Can you work these out from the model? Positions are in its coordinate system, mm. A direction names the side the tool comes from. Coordinates: 2 decimals unless noted, no trailing zeros. Write each loop counter-clockwise with the first axis right and the second up, starting at its lowest first coordinate (ties: lowest second). Pieces come first, ordered by that corner, then holes. Notation, with made-up numbers: (22, 32.25) - (66, 32.25) arc R17 cw to (66, 38.25) - close; hole circle Ø8 at (63, 63.25). An arc over 180 degrees is marked (long way). Use one line per item in the form item = value. Start each with the question number.
(1) Thinking about a two-plate mould opening in Z: for faces 1 (the face through (1, -54.6, -2)), 2 (the face through (-6.31, 11.71, 20.03)), 3 (the face through (0.04, -16.68, -17.78)), which applies, pulls with the +Z half, pulls with the -Z half, needs draft (parallel to the pull), parting line crosses it, or undercut?
(2) If we section it at A-A on y = 4: Please give me the cut outline in (x, z).
(3) If we section it at B-B on y = -44.6: Please give me the cut outline in (x, z).
(4) On a 3-axis mill with a long thin cutter (end or side, diameter ignored), from which of +Z, -Z, +X, -X, +Y, -Y can I reach the whole of each face in a straight line? I mean faces 4 (the face through (-1.216, -51.558, -1.115)), 5 (the face through (0, 16, 11)), 6 (the face through (2, -44, 4)). Say none if no direction works.
(5) For pin 1 Ø5 at (x, y) = (-1, -46) entering from +Z; pin 2 Ø4 at (x, z) = (-17.5, 0) entering from -Y; pin 3 Ø1.8 at (x, y) = (0, -44.6) entering from -Z; pin 4 Ø3 at (x, y) = (2, 27) entering from +Z, each with a flat end and sliding along its axis, tell me the tip position at first contact or that it passes through.
(6) If I drill on probe 1 along Y at (x, z) = (-14.5, -8.5); probe 2 along Y at (x, z) = (-5.5, -6.5); probe 3 along Y at (x, z) = (-8.5, 19), over which ranges is the centre line in solid material (lowest first)? Write a range as from..to.
```python
from build123d import *

# Parameters (mm, degrees)
SKETCH_2_W               = 28
SKETCH_2_H               = 4.5
CUT_EXTRUDE_1_DEPTH      = 10
EXTRUDE_1_DEPTH          = 15
HOLE_WIZARD_M3_1_D       = 2.5
HOLE_WIZARD_M3_1_DEPTH   = 4
HOLE_WIZARD_M3_1_TIP     = 0.751075774
CUT_EXTRUDE_START        = -20
CUT_EXTRUDE_2_DEPTH      = 20
HOLE_WIZARD_M4_1_D       = 3.3
HOLE_WIZARD_M4_1_DEPTH   = 10.1
HOLE_WIZARD_M4_1_TIP     = 0.991420021
CUT_EXTRUDE_3_DEPTH      = 64.617293246
CUT_EXTRUDE_3_DEPTH_BACK = 64.617293246
SKETCH_11_R              = 1.5
HOLE_WIZARD_M4_2_D       = 3.3
HOLE_WIZARD_M4_2_DEPTH   = 6
HOLE_WIZARD_M4_2_TIP     = 0.991420021


with BuildPart() as part:
    # 草图1 → 旋转1 (revolve)
    with BuildSketch(Plane.XY, mode=Mode.PRIVATE) as revolve_1_sk:
        Polygon((0, 0), (4.1, 0), (4.1, 6.7), (13.4, 6.7), (13.4, 8.7), (21, 8.7), (21, 10.2), (20, 10.2), (20, 11.2), (21, 11.2), (21, 12.2), (10, 12.2), (10, 13.2), (21, 13.2), (21, 20.4), (5, 20.4), (5, 21), (21, 21), (21, 34.7), (18.3, 38.7), (3.5, 38.7), (3.5, 43.7), (0, 43.7), align=None)
    revolve(revolve_1_sk.sketch.rotate(Axis((0, 43.7, 0), (0, -1, 0)), 90), axis=Axis((0, 43.7, 0), (0, -1, 0)))

    # 草图2 → 切除-拉伸1 (cut)
    with BuildSketch(Plane.XY.offset(21)):
        with Locations((0, 16.05)):
            Rectangle(SKETCH_2_W, SKETCH_2_H)
    extrude(amount=-CUT_EXTRUDE_1_DEPTH, mode=Mode.SUBTRACT)

    # 草图3 → 凸台-拉伸1 (add)
    with BuildSketch(Plane.XY.offset(11)):
        with BuildLine():
            Line((9.185056323, 18.053194417), (9.385056323, 18.053194417))
            ThreePointArc((9.385056323, 18.053194417), (11.385056323, 16.053194417), (9.385056323, 14.053194417))
            Line((9.385056323, 14.053194417), (9.185056323, 14.053194417))
            ThreePointArc((9.185056323, 14.053194417), (7.185056323, 16.053194417), (9.185056323, 18.053194417))
        make_face()
    extrude(amount=EXTRUDE_1_DEPTH)

    # M3 螺纹孔1
    with Locations(Plane(origin=(0, 38.7, 0), x_dir=(1, 0, 0), z_dir=(0, 1, 0))):
        with Locations((-6.5, 0), (6.5, 0)):
            Hole(HOLE_WIZARD_M3_1_D / 2, depth=HOLE_WIZARD_M3_1_DEPTH)
            with Locations((0, 0, -(HOLE_WIZARD_M3_1_DEPTH + HOLE_WIZARD_M3_1_TIP / 2))):  # 118° drill point
                Cone(0, HOLE_WIZARD_M3_1_D / 2, HOLE_WIZARD_M3_1_TIP, mode=Mode.SUBTRACT)

    # 草图7 → 旋转2 (revolve)
    with BuildSketch(Plane.XY, mode=Mode.PRIVATE) as revolve_2_sk:
        Polygon((0, -54.6), (5, -54.6), (5, -30.5), (8.275, -30.5), (8.275, -29.6), (13, -29.6), (13, -27.6), (21, -27.6), (21, 8.7), (0, 8.7), align=None)
    revolve(revolve_2_sk.sketch.rotate(Axis((0, 8.7, 0), (0, -1, 0)), 180), axis=Axis((0, 8.7, 0), (0, -1, 0)))

    # 草图8 → 切除-拉伸2 (cut)
    with BuildSketch(Plane.XZ.offset(54.6).offset(CUT_EXTRUDE_START)):
        with BuildLine():
            Line((-3, 4), (3, 4))
            ThreePointArc((3, 4), (0, 5), (-3, 4))
        make_face()
    extrude(amount=CUT_EXTRUDE_2_DEPTH, mode=Mode.SUBTRACT)

    # M4 螺纹孔1
    with Locations(Plane(origin=(0, -27.6, 0), x_dir=(-1, 0, 0), z_dir=(0, -1, 0))):
        with Locations((0, -17.5), (-17.5, 0), (0, 17.5), (17.5, 0)):
            Hole(HOLE_WIZARD_M4_1_D / 2, depth=HOLE_WIZARD_M4_1_DEPTH)
            with Locations((0, 0, -(HOLE_WIZARD_M4_1_DEPTH + HOLE_WIZARD_M4_1_TIP / 2))):  # 118° drill point
                Cone(0, HOLE_WIZARD_M4_1_D / 2, HOLE_WIZARD_M4_1_TIP, mode=Mode.SUBTRACT)

    # 草图11 → 切除-拉伸3 (cut, two sides: drawn at the far end of the back side and taken through both)
    with BuildSketch(Plane.XY.offset(4).offset(-CUT_EXTRUDE_3_DEPTH_BACK)):
        with Locations((0, -44.6)):
            Circle(SKETCH_11_R)
    extrude(amount=CUT_EXTRUDE_3_DEPTH + CUT_EXTRUDE_3_DEPTH_BACK, mode=Mode.SUBTRACT)

    # M4 螺纹孔2
    with Locations(Plane(origin=(0, -54.6, 0), x_dir=(-1, 0, 0), z_dir=(0, -1, 0))):
        with Locations((0, 0)):
            Hole(HOLE_WIZARD_M4_2_D / 2, depth=HOLE_WIZARD_M4_2_DEPTH)
            with Locations((0, 0, -(HOLE_WIZARD_M4_2_DEPTH + HOLE_WIZARD_M4_2_TIP / 2))):  # 118° drill point
                Cone(0, HOLE_WIZARD_M4_2_D / 2, HOLE_WIZARD_M4_2_TIP, mode=Mode.SUBTRACT)


solid = part.part
```
Reported:
q1.face_1 = needs draft
q1.face_2 = parting line crosses it
q1.face_3 = undercut
q2.outline = circle Ø42 at (0, 0)
q3.outline = (-3, 4) arc R5 ccw to (-1.5, -4.77) - (-1.5, 4) - close; (1.5, -4.77) arc R5 ccw to (3, 4) - (1.5, 4) - close
q4.face_4 = -Y
q4.face_5 = +Z
q4.face_6 = +Z, +X, -X, -Y
q5.pin_1 = 4
q5.pin_2 = -27.6
q5.pin_3 = through
q5.pin_4 = 20.99
q6.probe_1 = -27.6..12.2, 13.2..20.4, 21..38.7
q6.probe_2 = -29.6..20.4, 21..38.7
q6.probe_3 = -27.6..10.2, 11.2..12.2, 13.2..13.8, 18.3..20.4, 21..34.97
